```python
from build123d import *

# Parameters (mm, degrees)
F0_W      = 44.395774
F0_H      = 40.661618
F1_DEPTH  = 25.4
F1_FACE_W = 44.395774
F1_FACE_H = 40.661618
F2_DEPTH  = 25.4
F3_T      = -7.62
F4_R      = 6.796933
F5_DEPTH  = 25.4
F5_FACE_R = 6.796933
F6_DEPTH  = 50.8


with BuildPart() as f1:
    # F0 (on Top) → F1 (new body)
    with BuildSketch(Plane.XY):
        Rectangle(F0_W, F0_H)
    extrude(amount=F1_DEPTH)

    # F1_face (on face) → F2 (join)
    with BuildSketch(Plane(origin=(0, 0, 0), x_dir=(1, 0, 0), z_dir=(0, 0, -1))):
        Rectangle(F1_FACE_W, F1_FACE_H)
    extrude(amount=F2_DEPTH)

    # F3
    f3_openings = [f1.faces().sort_by_distance(p)[0] for p in [
        (0, -20.330809, 0),
        (0, 0, 25.4),
    ]]
    offset(amount=F3_T, openings=f3_openings)

    # F4 (on face) → F5 (join)
    with BuildSketch(Plane.YZ.offset(22.197887)):
        Circle(F4_R)
    extrude(amount=-F5_DEPTH)

    # F5_face (on face) → F6 (join)
    with BuildSketch(Plane(origin=(-3.202113, 0, 0), x_dir=(0, 1, 0), z_dir=(-1, 0, 0))):
        Circle(F5_FACE_R)
    extrude(amount=-F6_DEPTH)


solid = f1.part
```
Can you work these out from the model? Positions are in its coordinate system, mm. A direction names the side the tool comes from. Coordinates: 2 decimals unless noted, no trailing zeros. Order: outer loops, then holes, each group sorted by start corner. A loop starts at its lowest first (then second) coordinate and runs counter-clockwise, first axis right, second up.
1. If we section it at D-D (x = -12): Please give me the cut outline in (y, z).
2. Thinking about a two-plate mould opening in Y: for faces 1 (the face through (0, 12.711, 4)), 2 (the face through (0, 20.331, 0)), 3 (the face through (-3.202, 0, 0)), which applies, +Y half, -Y half, draft (parallel to the pull), parting line (faces both ways), or undercut?
3. If we section it at B-B (z = 0): Please give me the cut outline in (x, y), then the cut area to 3 significant figures.
4. I'm going to push flat-ended pins straight in: pin 1 (14.5 mm diameter, centred on x = 0.5, y = -9.5, fed in from +Z); pin 2 (1.5 mm diameter, centred on x = 14.5, y = -7.5, fed in from +Z); pin 3 (4 mm diameter, centred on y = -1, z = 13, fed in from +X); pin 4 (2 mm diameter, centred on x = 12.5, z = -2.5, fed in from -Y). Where does each tip first touch, or does it pass through?
5. For faces 4 (the face through (-14.578, -4, 4)), 5 (the face through (5.81, 3.14, -6.03)), 6 (the face through (22.198, -5, 6)), which set-ups out of +Z, -Z, +X, -X, +Y, -Y let a thin tool reach every point of the face, with its end or its side?
6. If we section it at A-A (x = 5): Please give me the cut outline in (y, z), then the cut area to 3 significant figures.
7. I need wall thicknesses on line 1 (X direction, y = -1, z = -3); line 2 (X direction, y = 0, z = 8.5); line 3 (Y direction, x = -12.5, z = 22.5). Which ranges of each line are inside material? Lowest first, please.
8. If we section it at C-C (y = -15): Please give me the cut outline in (x, z).
Entries:
1. outline: (-20.33, -25.4) - (20.33, -25.4) - (20.33, 25.4) - (12.71, 25.4) - (12.71, -17.78) - (-20.33, -17.78) - close
2. face 1: undercut
2. face 2: +Y half
2. face 3: draft
3. outline: (-22.2, -20.33) - (-14.58, -20.33) - (-14.58, 12.71) - (14.58, 12.71) - (14.58, 6.8) - (-3.2, 6.8) - (-3.2, -6.8) - (14.58, -6.8) - (14.58, -20.33) - (22.2, -20.33) - (22.2, -6.8) - (47.6, -6.8) - (47.6, 6.8) - (22.2, 6.8) - (22.2, 20.33) - (-22.2, 20.33) - close
3. area: 1,430 mm2
4. pin 1: stops at z = 6.41
4. pin 2: stops at z = 25.4
4. pin 3: stops at x = 22.2
4. pin 4: stops at y = -6.63
5. face 4: +Z, -Y
5. face 5: none
5. face 6: +X
6. outline: (-20.33, -25.4) - (20.33, -25.4) - (20.33, 25.4) - (12.71, 25.4) - (12.71, -17.78) - (-20.33, -17.78) - close; circle Ø13.59 at (0, 0)
6. area: 784 mm2
7. line 1: x = -22.2 to -14.58, -3.2 to 47.6
7. line 2: x = -22.2 to -14.58, 14.58 to 22.2
7. line 3: y = 12.71 to 20.33
8. outline: (-22.2, -25.4) - (22.2, -25.4) - (22.2, 25.4) - (14.58, 25.4) - (14.58, -17.78) - (-14.58, -17.78) - (-14.58, 25.4) - (-22.2, 25.4) - close
